Autodesk Inventor part; units mm, degrees
ref_plane "YZ Plane" through (0, 0, 0) normal (1, 0, 0) x (0, 1, 0)
ref_plane "XZ Plane" through (0, 0, 0) normal (0, 1, 0) x (-1, 0, 0)
ref_plane "XY Plane" through (0, 0, 0) normal (0, 0, 1) x (1, 0, 0)
sketch "Sketch1" plane through (0, 0, 0) normal (0, 1, 0) x (-1, 0, 0)
  line L0 (289.4755, 0) -> (-215.021, 0)
  line L1 (0, 324.0308) -> (0, -320.0636)
  circle A0 centre (0, 0) radius 10 construction
  line L2 (17.3205, 10) -> (50, -46.6025)
  line L3 (50, -46.6025) -> (0, -46.6025) construction
  line L4 (-17.3205, 10) -> (-50, -46.6025)
  line L5 (-50, -46.6025) -> (0, -46.6025) construction
  arc A1 (17.3205, 10) -> (-17.3205, 10) centre (0, 0) ccw
  line L6 (50, -46.6025) -> (50, -66.6025)
  line L7 (50, -66.6025) -> (-50, -66.6025)
  line L8 (-50, -66.6025) -> (-50, -46.6025)
  point P0 (0, 40)
  dimension "d0" = 20
  dimension "d1" = 50
  dimension "d2" = 60
  dimension "d3" = 40
  dimension "d4" = 20
  dimension "d5" = 20
extrude "Extrusion1" add sketch "Sketch1" along normal mid plane 360
sketch "Sketch2" plane through (0, 0, 0) normal (0, 1, 0) x (-1, 0, 0)
  line L0 (0, 66.6254) -> (0, -94.0572)
  line L1 (109.0661, 0) -> (-97.6998, 0)
  line L2 (0, -6) -> (150, -6)
  line L3 (150, -6) -> (150, -16)
  line L4 (150, -16) -> (140, -16)
  line L5 (140, -16) -> (50, -106)
  line L6 (50, -106) -> (0, -106)
  line L7 (0, -106) -> (0, -6)
  point P0 (0, 0)
  point P1 (0, -94.0572)
  dimension "d8" = 150
  dimension "d9" = 12
  dimension "d10" = 135
  dimension "d11" = 50
  dimension "d12" = 100
  dimension "d13" = 10
revolve "Revolution1" add sketch "Sketch2" angle 360 about axis through (0, 0, 66.6254) along (0, 0, -1)
sketch "Sketch3" plane through (0, 0, -6) normal (0, 0, 1) x (1, 0, 0)
  circle A0 centre (0, 0) radius 163
  dimension "d15" = 326
extrude "Extrusion2" cut sketch "Sketch3" along normal blind 360
sketch "Sketch4" plane through (0, 180, 0) normal (0, 1, 0) x (1, 0, 0)
  circle A0 centre (0, 0) radius 8
  dimension "d18" = 16
extrude "Extrusion3" add sketch "Sketch4" along normal blind 12
mirror "Mirror1" about plane through (0, 0, 0) normal (0, 1, 0) of "Extrusion3"
chamfer "Chamfer1" distance 2 angle 45 2 edges at (-150, 0, -6) (-150, 0, -16)
properties part number "B_axis"
Verification items for the finished model (mm, model axes). A direction names the side the tool comes from. Coordinates: 2 decimals unless noted, no trailing zeros. Write each loop counter-clockwise with the first axis right and the second up, starting at its lowest first coordinate (ties: lowest second). Pieces come first, ordered by that corner, then holes. Notation, with made-up numbers: M 23.5,-36.75 L 34.5,-36.75 A14 cw 34.5,-17.75 Z; hole C 22.25,76.25 d6. An arc over 180 degrees is marked long. Answer as a JSON object with one key per item and string values. Group by question number.
(1) Gauge pin test, flat ends, axial feed: pin 1 (6 mm diameter, centred on x = 67.5, z = -31.5, fed in from +Y); pin 2 (12 mm diameter, centred on x = 9.5, z = -52.5, fed in from -Y); pin 3 (16 mm diameter, centred on y = 119.5, z = -53, fed in from -X). Record the tip position at first contact, or that the pin passes through.
(2) Tool access check on faces 1 (the face through (-50, 138, -56)), 2 (the face through (50, 126, -57)), 3 (the face through (0, -171, 20)), 4 (the face through (-50, -128, -56)), 5 (the face through (-1.73, -185.92, 7.81)). Record the directions out of +Z, -Z, +X, -X, +Y, -Y that give a thin tool (end or side, any length) a straight path to the whole face; none if there is none.
(3) Cross-section at B-B, the plane y = 0. Record the cut outline in (x, z), and give its area (3 significant figures).
(4) Material ranges on line 1 (Z direction, x = -4.5, y = -153); line 2 (Y direction, x = -12, z = -43); line 3 (Z direction, x = 97, y = -76.5), recorded low to high.
(5) Cross-section at D-D, the plane z = -94.5. Record the cut outline in (x, y), and give its area (3 significant figures).
(6) Release check for a two-part mould opening along Y. For faces 6 (the face through (149.97, 2.92, -11.07)), 7 (the face through (50, -128, -57)), 8 (the face through (0, 163, 4)), 9 (the face through (1, -180, -32)) record: +Y half, -Y half, draft (parallel to the pull), parting line (faces both ways), or undercut.
(7) Cross-section at A-A, the plane z = 0. Record the cut outline in (x, y).
(8) Cross-section at C-C, the plane x = 0. Record the cut outline in (y, z), and give its area (3 significant figures).
Reply:
{
 "1": {"pin 1": "y = 108.62", "pin 2": "y = -180", "pin 3": "x = -50"},
 "2": {"face 1": "-Z, -X, +Y", "face 2": "-Z, +X, +Y", "face 3": "+Z, +Y, -Y", "face 4": "-Z, -X, -Y", "face 5": "-Y"},
 "3": {"outline": "M -150,-14 L -148,-16 L -140,-16 L -50,-106 L 50,-106 L 140,-16 L 150,-16 L 150,-6 L -148,-6 L -150,-8 Z", "area": "20,100 mm²"},
 "4": {"line 1": "-66.6 to -6", "line 2": "-180 to 180", "line 3": "-32.46 to -6"},
 "5": {"outline": "C 0,0 d123", "area": "11,900 mm²"},
 "6": {"face 6": "parting line", "face 7": "draft", "face 8": "undercut", "face 9": "-Y half"},
 "7": {"outline": "M -23.09,-180 L -8,-180 L -8,-192 L 8,-192 L 8,-180 L 23.09,-180 L 23.09,-161.36 A163 cw -23.09,-161.36 Z; M -23.09,161.36 A163 cw 23.09,161.36 L 23.09,180 L 8,180 L 8,192 L -8,192 L -8,180 L -23.09,180 Z"},
 "8": {"outline": "M -192,-8 L -180,-8 L -180,-66.6 L -89.4,-66.6 L -50,-106 L 50,-106 L 89.4,-66.6 L 180,-66.6 L 180,-8 L 192,-8 L 192,8 L 180,8 L 180,20 L 163,20 L 163,-6 L -163,-6 L -163,20 L -180,20 L -180,8 L -192,8 Z", "area": "28,600 mm²"}
}
